```python
from build123d import *

# Parameters (mm, degrees)
SKETCH_1_R          = 1.5
EXTRUDE_1_DEPTH     = 16
SKETCH_2_R          = 1.35
CUT_EXTRUDE_1_DEPTH = 10
CUT_EXTRUDE_2_DEPTH = 33
EXTRUDE_2_DEPTH     = 16
SKETCH_5_R          = 1.5
CUT_EXTRUDE_3_DEPTH = 24
SKETCH_7_R          = 1.8
CUT_EXTRUDE_5_DEPTH = 10


with BuildPart() as part:
    # 草图1 → 凸台-拉伸1 (new body)
    with BuildSketch(Plane.XY):
        with BuildLine():
            Line((1.126380295, 5.893323971), (37.220974686, -1.005370225))
            Line((37.220974686, -1.005370225), (63.227984205, -49.979924472))
            Line((63.227984205, -49.979924472), (112.538061605, -75))
            Line((112.538061605, -75), (53.330616959, -72.391905084))
            Line((53.330616959, -72.391905084), (49.915441771, -64.88738307))
            Line((49.915441771, -64.88738307), (26.682733599, -13.835720919))
            Line((26.682733599, -13.835720919), (-1.643050648, -5.77064854))
            ThreePointArc((-1.643050648, -5.77064854), (-5.837705093, 1.386073321), (1.126380295, 5.893323971))
        make_face()
        Circle(SKETCH_1_R, mode=Mode.SUBTRACT)
    extrude(amount=EXTRUDE_1_DEPTH)

    # 草图2 → 切除-拉伸1 (cut)
    with BuildSketch(Plane(origin=(-3.079413203, -69.907036606, 0), x_dir=(0.9990312032291818, -0.044007442262116094, 0), z_dir=(-0.044007442262116094, -0.9990312032291818, 0))):
        with Locations((66, 8)):
            Circle(SKETCH_2_R)
        with Locations((102, 8)):
            Circle(SKETCH_2_R)
        with Locations((84, 8)):
            Circle(SKETCH_2_R)
    extrude(amount=-CUT_EXTRUDE_1_DEPTH, mode=Mode.SUBTRACT)

    # 草图3 → 切除-拉伸2 (cut)
    with BuildSketch(Plane.XY.offset(16)):
        Polygon((26.682733599, -13.835720919), (54.911117554, -72.461526322), (53.330616959, -72.391905084), align=None)
    extrude(amount=-CUT_EXTRUDE_2_DEPTH, mode=Mode.SUBTRACT)

    # 草图4 → 凸台-拉伸2 (add)
    with BuildSketch(Plane.XY.offset(16)):
        Polygon((44.895473102, -51.660646486), (37.739057149, -36.797923572), (27.624132339, -36.797923572), (27.532134383, -51.660646486), align=None)
    extrude(amount=-EXTRUDE_2_DEPTH)

    # 草图5 → 切除-拉伸3 (cut)
    with BuildSketch(Plane.XY.offset(16)):
        with Locations((47.911117554, -40.461526322)):
            Circle(SKETCH_5_R)
    extrude(amount=-CUT_EXTRUDE_3_DEPTH, mode=Mode.SUBTRACT)

    # 草图7 → 切除-拉伸5 (cut)
    with BuildSketch(Plane(origin=(27.85083871, -0.172392383, 0), x_dir=(0, 0, 1), z_dir=(-0.9999808434581536, 0.006189726708003564, 0))):
        with Locations(Location((8, -44.015961614, 0), (0, 0, 270))):
            Circle(SKETCH_7_R)
    extrude(amount=-CUT_EXTRUDE_5_DEPTH, mode=Mode.SUBTRACT)


solid = part.part
```
Part model, mm, in its own coordinate system. A direction names the side the tool comes from. Give positions to 0.01 mm unless a question says otherwise; leave off trailing zeros. Order: outer loops, then holes, each group sorted by start corner. A loop starts at its lowest first (then second) coordinate and runs counter-clockwise, first axis right, second up. Notation, with made-up numbers: M 53,22 L 76,22 A20 cw 76,57 Z; hole C -29,5 d9. An arc over 180 degrees is marked long. Use a Markdown table: item, result. Add a question column.
(1) 3-axis set-ups, long thin cutter, end or side, ignore diameter. For faces 4 (the face through (49.833, -61.915, 8.112)), 5 (the face through (81.26, -63.613, 8.019)): which of +Z, -Z, +X, -X, +Y, -Y reach the whole face in a straight line?
(2) Drop flat-ended pins along their axis: P1, Ø6, axis at x = 6, z = 5, coming from the +Y side; P2, Ø5, axis at x = 31.5, z = 9, coming from the +Y side; P3, Ø8, axis at x = 89.5, z = 11, coming from the +Y side; P4, Ø2.5, axis at x = 47.91, y = -40.46, coming from the +Z side. Give the stop position or say it passes through.
(3) Saw through at C-C, the plane y = -3. Give the cut face in (x, z).
(4) Mould opens along Z. For faces 1 (the face through (49, -37, 16)), 2 (the face through (32.503, -45.049, 6.403)), 3 (the face through (87.538, -62.315, 7.888)) say: +Z half, -Z half, draft (parallel to the pull), parting line (faces both ways), or undercut.
(5) Saw through at A-A, the plane z = 4. Give the cut face in (x, y).
(6) Saw through at B-B, the plane x = 90. Give the cut face in (y, z), and give its area (3 significant figures).
(7) Probe line 1 along Y through (x, z) = (0, 11); line 2 along Y through (x, z) = (24, 11.5); line 3 along Y through (x, z) = (54, 1). List the from-to ranges inside material, lowest first. Write a range as [from, to].
(8) Saw through at D-D, the plane y = -66. Give the number of separate pieces and of enclosed holes in the cut face, and give its area (3 significant figures).
Answer key:
| question | item | result |
|---|---|---|
| 1 | face 4 | +Z, -Z, -X, -Y |
| 1 | face 5 | none |
| 2 | P1 | y = 5.54 |
| 2 | P2 | y = 0.57 |
| 2 | P3 | y = -61.28 |
| 2 | P4 | through |
| 3 | outline | M -5.2,0 L 38.28,0 L 38.28,16 L -5.2,16 Z |
| 4 | face 1 | +Z half |
| 4 | face 2 | undercut |
| 4 | face 3 | draft |
| 5 | outline | M -1.64,-5.77 L 26.68,-13.84 L 37.74,-36.8 L 27.62,-36.8 L 27.53,-51.66 L 44.9,-51.66 L 54.91,-72.46 L 112.54,-75 L 63.23,-49.98 L 37.22,-1.01 L 1.13,5.89 A6 ccw Z; hole C 0,0 d3; hole C 47.91,-40.46 d3 |
| 6 | outline | M -74.01,0 L -63.56,0 L -63.56,16 L -74.01,16 Z |
| 6 | area | 167 mm^2 |
| 7 | line 1 | [-6.24, -1.5], [1.5, 6] |
| 7 | line 2 | [-13.07, 1.52] |
| 7 | line 3 | [-70.57, -32.6] |
| 8 | separate pieces | 1 |
| 8 | enclosed holes | 2 |
| 8 | area | 677 mm^2 |
